from build123d import *

# Parameters (mm, degrees)
SKETCH1_R           = 1.575
BOSS_EXTRUDE1_DEPTH = 1.5875


with BuildPart() as part:
    # Sketch1 → Boss-Extrude1 (new body, symmetric)
    with BuildSketch(Plane.XY):
        Polygon((163, 71.825), (163, 75), (113, 75), (113, 71.825), (63, 71.825), (63, 75), (13, 75), (13, 71.825), (3.175, 71.825), (3.175, 50.825), (0, 50.825), (0, 29.825), (3.175, 29.825), (3.175, 8.825), (0, 8.825), (0, 0), (63, 0), (63, 8.825), (113, 8.825), (113, 0), (176, 0), (176, 8.825), (172.825, 8.825), (172.825, 29.825), (176, 29.825), (176, 50.825), (172.825, 50.825), (172.825, 71.825), align=None)
        with Locations((33.0875, 6.61875)):
            Circle(SKETCH1_R, mode=Mode.SUBTRACT)
        with Locations((142.9125, 7.2375)):
            Circle(SKETCH1_R, mode=Mode.SUBTRACT)
    extrude(amount=BOSS_EXTRUDE1_DEPTH, both=True)


solid = part.part
Input: part model. Units: mm. Frame: model coordinates. A direction names the side the tool comes from. Round coordinates to 2 decimals unless told otherwise and drop trailing zeros. Order: outer loops, then holes, each group sorted by start corner. A loop starts at its lowest first (then second) coordinate and runs counter-clockwise, first axis right, second up.
1. Cut plane A-A, the plane z = 1.1. State how many separate pieces and enclosed holes the cut face has, then the cut area to 3 significant figures.
The answers:
separate pieces: 1
enclosed holes: 2
area: 12,200 mm2
2. Mould query, pull axis X, two halves, no side actions, for faces 6 (the face through (176, 40, 0)), 7 (the face through (144.415, 7.711, -0.022)), 8 (the face through (174, 50.825, 0)). Classes: released by +X, released by -X, zero draft, split by the parting line, or undercut.
The answers:
face 6: released by +X
face 7: undercut
face 8: zero draft
3. Material intervals for line 1 (X direction, y = 65.5, z = -0.7) (3 decimals); line 2 (Y direction, x = 86, z = -0.6) (3 decimals); line 3 (Y direction, x = 165.5, z = -0.25) (3 decimals), sorted ascending.
The answers:
line 1: x = 3.175 to 172.825
line 2: y = 8.825 to 71.825
line 3: y = 0 to 71.825
4. Cut plane C-C, the plane y = 66.5. Output: boundary loops of the cut face in (x, z) (1 decimal).
The answers:
outline: (3.2, -1.6) - (172.8, -1.6) - (172.8, 1.6) - (3.2, 1.6) - close
5. Cut plane B-B, the plane x = 102.5. Output: boundary loops of the cut face in (y, z) (1 decimal).
The answers:
outline: (8.8, -1.6) - (71.8, -1.6) - (71.8, 1.6) - (8.8, 1.6) - close
6. Pin query (flat end, axial travel): P1, Ø1.6, axis at y = 58.5, z = 0.5, coming from the +X side (3 decimals); P2, Ø1, axis at y = 73, z = 0, coming from the +X side; P3, Ø1, axis at y = 73, z = -0.5, coming from the -X side; P4, Ø4, axis at x = 33.09, y = 6.62, coming from the -Z side. Return the tip coordinate at first contact, or that it passes through.
The answers:
P1: stops at x = 172.825
P2: stops at x = 163
P3: stops at x = 13
P4: stops at z = -1.59
7. Set-up query: faces 1 (the face through (13, 73, 0)), 2 (the face through (174, 29.825, 0)), 3 (the face through (3.175, 19, 0)), 4 (the face through (88, 8.825, 0)), 5 (the face through (172.825, 61, 0)). Return all of +Z, -Z, +X, -X, +Y, -Y with unobstructed straight access to the full face (end or side cutting, diameter ignored); none if empty.
The answers:
face 1: +Z, -Z, -X, +Y
face 2: +Z, -Z, +X
face 3: +Z, -Z, -X
face 4: +Z, -Z, -Y
face 5: +Z, -Z, +X, +Y
